```python
from build123d import *

# Parameters (mm, degrees)
F0_R     = 12.7
F1_DEPTH = 38.1
F2_W     = 38.1
F2_H     = 25.4
F2_H_2   = 50.8
F3_DEPTH = 88.9
F4_R     = 5.08
F5_R     = 1.27


with BuildPart() as f1:
    # F0 (on Right) → F1 (new body, symmetric)
    with BuildSketch(Plane.YZ):
        with BuildLine():
            Line((152.4, 25.4), (152.4, 38.1))
            Line((152.4, 38.1), (-152.4, 38.1))
            Line((-152.4, 38.1), (-152.4, 25.4))
            ThreePointArc((-152.4, 25.4), (-177.8, 0), (-152.4, -25.4))
            Line((-152.4, -25.4), (-152.4, -38.1))
            Line((-152.4, -38.1), (152.4, -38.1))
            Line((152.4, -38.1), (152.4, -25.4))
            ThreePointArc((152.4, -25.4), (177.8, 0), (152.4, 25.4))
        make_face()
        with Locations((-152.4, 0)):
            Circle(F0_R, mode=Mode.SUBTRACT)
        with Locations((152.4, 0)):
            Circle(F0_R, mode=Mode.SUBTRACT)
    extrude(amount=F1_DEPTH, both=True)

    # F2 (on face) → F3 (cut)
    with BuildSketch(Plane.XY.offset(38.1)):
        with Locations((0, 165.1)):
            Rectangle(F2_W, F2_H)
        with Locations((0, 127)):
            Rectangle(F2_W, F2_H_2)
        with Locations((0, -127)):
            Rectangle(F2_W, F2_H_2)
        with Locations((0, -165.1)):
            Rectangle(F2_W, F2_H)
    extrude(amount=-F3_DEPTH, mode=Mode.SUBTRACT)

    # F4
    f4_edges = [f1.edges().sort_by_distance(p)[0] for p in [
        (28.575, 152.4, -38.1),
        (-28.575, 152.4, -38.1),
        (-28.575, 152.4, 38.1),
        (28.575, 152.4, 38.1),
        (28.575, -152.4, -38.1),
        (-28.575, -152.4, -38.1),
        (28.575, -152.4, 25.4),
        (-28.575, -152.4, 38.1),
    ]]
    fillet(f4_edges, radius=F4_R)

    # F5
    f5_edges = [f1.edges().sort_by_distance(p)[0] for p in [
        (19.05, 101.6, 0),
        (-19.05, 101.6, 0),
        (19.05, -101.6, 0),
        (-19.05, -101.6, 0),
    ]]
    fillet(f5_edges, radius=F5_R)


solid = f1.part
```
Read the model definition and answer for the solid it produces. Units are mm, in the model's axes. A direction names the side the tool comes from. Give positions to 0.01 mm unless a question says otherwise; leave off trailing zeros. Loops run counter-clockwise (first coordinate to the right, second up) from the corner with the lowest first, then second, coordinate; pieces in that order, holes last.
Item 1: Find the intervals of material crossed by line 1 along Y through (x, z) = (25, 0); line 2 along X through (y, z) = (102.5, 22); line 3 along Y through (x, z) = (-33, 29.5), in increasing order.
Item 2: Each of these flat-tipped pins is pushed along its axis until it touches: pin 1 Ø4 at (x, z) = (29.5, -28.5) entering from -Y; pin 2 Ø6 at (x, z) = (-30, 28.5) entering from +Y; pin 3 Ø18 at (x, z) = (9, -6) entering from -Y; pin 4 Ø5 at (x, y) = (16.5, -119.5) entering from -Z. Where does it stop, or does it pass through?
Item 3: The part is cut by section C-C (y = -115). Write down the section's boundary in (x, z), and give its area (3 significant figures).
Item 4: The part is cut by section B-B (z = 0). Give the number of separate pieces and of enclosed holes in the cut face, and give its area (3 significant figures).
Item 5: The part is cut by section D-D (y = 143). Write down the section's boundary in (x, z).
Item 6: For faces 1 (the flat face through (-28, -152.4, 29)), 2 (the flat face through (29, 152.4, -29)), 3 (the flat face through (19.05, -133, 1)), 4 (the flat face through (29, -152.4, 34)), determine the directions among +Z, -Z, +X, -X, +Y, -Y from which every point of the face is accessible in a straight line to the end or side of a thin tool.
Item 7: The part is cut by section A-A (x = -23). Write down the section's boundary in (y, z), and give its area (3 significant figures).
Item 8: The mould has two halves that part along X. Classify faces 5 (the cylindrical face through (28.442, -165.088, 0.558)), 6 (the flat face through (-19.05, 133, 1)), 7 (the flat face through (-38.1, -2, 1)): released by +X, released by -X, zero draft, split by the parting line, or undercut.
Taken from the geometry:
1. line 1: y = -177.8 to -165.1, -139.7 to 139.7, 165.1 to 177.8
1. line 2: x = -38.1 to -18.99, 18.99 to 38.1
1. line 3: y = -152.4 to 152.4
2. pin 1: stops at y = -152.4
2. pin 2: stops at y = 152.4
2. pin 3: stops at y = -101.62
2. pin 4: passes through
3. outline: (-38.1, -38.1) - (-19.05, -38.1) - (-19.05, 38.1) - (-38.1, 38.1) - close; (19.05, -38.1) - (38.1, -38.1) - (38.1, 38.1) - (19.05, 38.1) - close
3. area: 2,900 mm2
4. separate pieces: 5
4. enclosed holes: 0
4. area: 19,400 mm2
5. outline: (-38.1, -38.1) - (-19.05, -38.1) - (-19.05, -8.54) - (-38.1, -8.54) - close; (-38.1, 8.54) - (-19.05, 8.54) - (-19.05, 38.1) - (-38.1, 38.1) - close; (19.05, -38.1) - (38.1, -38.1) - (38.1, -8.54) - (19.05, -8.54) - close; (19.05, 8.54) - (38.1, 8.54) - (38.1, 38.1) - (19.05, 38.1) - close
6. face 1: +Z, -X, -Y
6. face 2: -Z, +X, -X, +Y
6. face 3: +Z, -Z, -Y
6. face 4: +Z, +X, -X, -Y
7. outline: (-152.4, -33.02) arc R5.08 ccw to (-147.32, -38.1) - (147.32, -38.1) arc R5.08 ccw to (152.4, -33.02) - (152.4, -25.4) arc R25.4 ccw to (152.4, 25.4) - (152.4, 33.02) arc R5.08 ccw to (147.32, 38.1) - (-147.32, 38.1) arc R5.08 ccw to (-152.4, 33.02) - (-152.4, 25.4) arc R25.4 ccw to (-152.4, -25.4) - close; hole circle Ø25.4 at (-152.4, 0); hole circle Ø25.4 at (152.4, 0)
7. area: 24,200 mm2
8. face 5: zero draft
8. face 6: undercut
8. face 7: released by -X
